Autodesk Inventor part; units mm, degrees
ref_plane "YZ Plane" through (0, 0, 0) normal (1, 0, 0) x (0, 1, 0)
ref_plane "XZ Plane" through (0, 0, 0) normal (0, 1, 0) x (-1, 0, 0)
ref_plane "XY Plane" through (0, 0, 0) normal (0, 0, 1) x (1, 0, 0)
sketch "Sketch1" plane through (0, 0, 0) normal (1, 0, 0) x (0, 1, 0)
  line L0 (10.812, 12.057) -> (-14.132, 12.057)
  line L1 (-14.132, 12.057) -> (-14.132, -3.8443)
  line L2 (-14.132, -3.8443) -> (10.812, -3.8443)
  line L3 (10.812, -3.8443) -> (10.812, 12.057)
  point P0 (0, 0)
extrude "Extrusion1" add sketch "Sketch1" along normal blind 17.78
sketch "Sketch2" plane through (17.78, 0, 0) normal (1, 0, 0) x (0, 0, -1)
  line L0 (-8.2866, -8.1756) -> (1.1098, -8.1756)
  line L1 (1.1098, -8.1756) -> (1.1098, -12.3189)
  line L2 (1.1098, -12.3189) -> (-8.2866, -12.3189)
  line L3 (-8.2866, -12.3189) -> (-8.2866, -8.1756)
  line L4 (-8.2866, -1.4428) -> (1.1098, -1.4428)
  line L5 (1.1098, -1.4428) -> (1.1098, -5.734)
  line L6 (1.1098, -5.734) -> (-8.2866, -5.734)
  line L7 (-8.2866, -5.734) -> (-8.2866, -1.4428)
  point P0 (0, 0)
extrude "Extrusion2" cut sketch "Sketch2" against normal blind 10.16
sketch "Sketch3" plane through (0, 0, 0) normal (-1, 0, 0) x (0, 0, 1)
  line L0 (8.2866, -12.3189) -> (8.2866, -8.1756)
  line L1 (0.5236, -9.8392) -> (8.2866, -9.8392)
  line L2 (8.2866, -9.8392) -> (8.2866, -11.7154)
  line L3 (8.2866, -11.7154) -> (0.5236, -11.7154)
  line L4 (0.5236, -11.7154) -> (0.5236, -9.8392)
  point P0 (0, 0)
extrude "Extrusion3" cut sketch "Sketch3" against normal blind 25.4
Can you work these out from the model? Positions are in its coordinate system, mm. A direction names the side the tool comes from. Coordinates: 2 decimals unless noted, no trailing zeros. Order: outer loops, then holes, each group sorted by start corner. A loop starts at its lowest first (then second) coordinate and runs counter-clockwise, first axis right, second up. Notation, with made-up numbers: (81.5, 8) - (128.5, 8) arc R13 cw to (128.5, 19) - close; hole circle Ø7 at (23.25, -26). An arc over 180 degrees is marked (long way). Answer as a JSON object with one key per item and string values. Group by question number.
Q1. Imagine slicing it at A-A (z = 1.25). Please give me the cut outline in (x, y), and give its area (3 significant figures).
Q2. Imagine slicing it at B-B (x = 4.25). Please give me the cut outline in (y, z).
Q3. Will this pin go through, and if not, where does the flat tip stop? P1, Ø1.2, axis at y = -10, z = 3, coming from the +X side.
Q4. On a 3-axis mill with a long thin cutter (end or side, diameter ignored), from which of +Z, -Z, +X, -X, +Y, -Y can I reach the whole of each face in a straight line? I mean faces 1 (the face through (13, -4, 8.287)), 2 (the face through (4, -11.715, 4)), 3 (the face through (9, -14.132, 4)). Say none if no direction works.
Q5. Imagine slicing it at D-D (y = -4.75). Please give me the cut outline in (x, z).
Q6. Imagine slicing it at C-C (x = 10). Please give me the cut outline in (y, z).
Q7. I need wall thicknesses on line 1 (Y direction, x = 10, z = -0.5); line 2 (Z direction, x = 4.5, y = -10.25); line 3 (X direction, y = -8.5, z = 5). Which ranges of each line are inside material? Lowest first, please. Write a range as from..to.
Determined:
{
 "1": {"outline": "(0, -14.13) - (17.78, -14.13) - (17.78, -12.32) - (7.62, -12.32) - (7.62, -11.72) - (0, -11.72) - close; (0, -9.84) - (7.62, -9.84) - (7.62, -8.18) - (17.78, -8.18) - (17.78, -5.73) - (7.62, -5.73) - (7.62, -1.44) - (17.78, -1.44) - (17.78, 10.81) - (0, 10.81) - close", "area": "344 mm2"},
 "2": {"outline": "(-14.13, -3.84) - (10.81, -3.84) - (10.81, 12.06) - (-14.13, 12.06) - close; hole (-11.72, 0.52) - (-9.84, 0.52) - (-9.84, 8.29) - (-11.72, 8.29) - close"},
 "3": {"P1": "stops at x = 7.62"},
 "4": {"face 1": "+X", "face 2": "+X, -X", "face 3": "+Z, -Z, +X, -X, -Y"},
 "5": {"outline": "(0, -3.84) - (17.78, -3.84) - (17.78, -1.11) - (7.62, -1.11) - (7.62, 8.29) - (17.78, 8.29) - (17.78, 12.06) - (0, 12.06) - close"},
 "6": {"outline": "(-14.13, -3.84) - (10.81, -3.84) - (10.81, 12.06) - (-14.13, 12.06) - close; hole (-12.32, -1.11) - (-8.18, -1.11) - (-8.18, 8.29) - (-12.32, 8.29) - close; hole (-5.73, -1.11) - (-1.44, -1.11) - (-1.44, 8.29) - (-5.73, 8.29) - close"},
 "7": {"line 1": "y = -14.13..-12.32, -8.18..-5.73, -1.44..10.81", "line 2": "z = -3.84..0.52, 8.29..12.06", "line 3": "x = 0..7.62"}
}
